Source: CAD feature listing. Evaluate the final solid. Frame: model axes, mm. Give positions to 0.01 mm unless a question says otherwise; leave off trailing zeros. Loops run counter-clockwise (first coordinate to the right, second up) from the corner with the lowest first, then second, coordinate; pieces in that order, holes last. Notation, with made-up numbers: (-12.75, 32.5) -> (28.25, 32.5) arc R35 cw to (28.25, 71.5) -> close; hole circle Ø11 at (-14, 82). An arc over 180 degrees is marked (long way). Answer as a JSON object with one key per item and string values. Group by question number.
from build123d import *

# Parameters (mm, degrees)
F1_W     = 258.840755
F1_H     = 209.543214
F2_DEPTH = 25.4
F3_DEPTH = 25.4
F4_W     = 239.790755
F4_H     = 196.843214
F5_DEPTH = 19.05


with BuildPart() as f2:
    # F1 (on Front) → F2 (new body)
    with BuildSketch(Plane.XZ):
        with Locations((20.0017, 0.897209)):
            Rectangle(F1_W, F1_H)
    extrude(amount=-F2_DEPTH)

    # F0 (on Front) → F3 (cut)
    with BuildSketch(Plane.XZ):
        Polygon((-88.651664, 86.055733), (-82.07436, 74.663833), (-88.651664, 63.271933), (-82.07436, 51.880033), (-88.651664, 40.488133), (-82.07436, 29.096233), (-88.651664, 17.704333), (-82.07436, 6.312433), (-88.651664, -5.079467), (-82.07436, -16.471367), (-88.651664, -27.863267), (-82.07436, -39.255167), (-88.651664, -50.647067), (-82.07436, -62.038967), (-88.651664, -73.430867), (-82.07436, -84.822767), (-68.5546, -84.810067), (-61.977295, -96.201967), (-48.074809, -96.201967), (-41.497504, -84.810067), (-29.09062, -84.810067), (-22.513315, -96.201967), (-8.610829, -96.201967), (-2.033524, -84.810067), (10.37336, -84.810067), (16.950665, -96.201967), (30.853151, -96.201967), (37.430456, -84.810067), (49.83734, -84.810067), (56.414645, -96.201967), (70.308445, -96.201967), (77.259713, -84.162367), (70.682409, -72.770467), (77.259713, -61.378567), (70.682409, -49.986667), (77.259713, -38.594767), (70.682409, -27.202867), (77.259713, -15.810967), (70.682409, -4.419067), (77.259713, 6.972833), (70.682409, 18.364733), (77.259713, 29.756633), (70.682409, 41.148533), (77.259713, 52.540433), (70.682409, 63.932333), (77.259713, 75.324233), (70.681266, 86.718775), (57.162446, 86.703433), (50.585141, 98.095333), (36.682655, 98.095333), (30.10535, 86.703433), (17.698466, 86.703433), (11.121161, 98.095333), (-2.781325, 98.095333), (-9.35863, 86.703433), (-21.765514, 86.703433), (-28.342819, 98.095333), (-42.252925, 98.095333), (-48.83023, 86.703433), (-61.237114, 86.703433), (-67.814419, 98.095333), (-81.700395, 98.095333), align=None)
    extrude(amount=-F3_DEPTH, mode=Mode.SUBTRACT)

    # F4 (on face) → F5 (cut)
    with BuildSketch(Plane(origin=(0, 25.4, 0), x_dir=(-1, 0, 0), z_dir=(0, 1, 0))):
        with Locations((-16.826699, 0.897209)):
            Rectangle(F4_W, F4_H)
    extrude(amount=-F5_DEPTH, mode=Mode.SUBTRACT)


solid = f2.part
(1) Section query A-A on x = -34. Return the cut outline in (y, z), plus the area to 3 significant figures.
(2) Mould query, pull axis X, two halves, no side actions, for faces 1 (the face through (74.02, 3.13, -78.55)), 2 (the face through (73.9, 3.1, -67.2)). Classes: pulls with the +X half, pulls with the -X half, needs draft (parallel to the pull), parting line crosses it, or undercut.
(3) Material intervals for line 1 (X direction, y = 16.5, z = 27); line 2 (Z direction, x = -33, y = 15.25); line 3 (Z direction, x = -76.5, y = 2), sorted ascending. Write a range as from..to.
(4) Section query B-B on z = 55.5. Return the cut outline in (x, y), plus the area to 3 significant figures.
(5) Section query D-D on x = 120. Return the cut outline in (y, z), plus the area to 3 significant figures.
(6) Section query C-C on y = 9.25. Return the cut outline in (x, z).
Result:
{
 "1": {"outline": "(0, -103.87) -> (25.4, -103.87) -> (25.4, -97.52) -> (6.35, -97.52) -> (6.35, -84.81) -> (0, -84.81) -> close; (0, 98.1) -> (6.35, 98.1) -> (6.35, 99.32) -> (25.4, 99.32) -> (25.4, 105.67) -> (0, 105.67) -> close", "area": "411 mm²"},
 "2": {"face 1": "undercut", "face 2": "undercut"},
 "3": {"line 1": "-109.42..-103.07, 136.72..149.42", "line 2": "-103.87..-97.52, 99.32..105.67", "line 3": "-103.87..-84.82, 98.1..105.67"},
 "4": {"outline": "(-109.42, 0) -> (-84.16, 0) -> (-84.16, 6.35) -> (-103.07, 6.35) -> (-103.07, 25.4) -> (-109.42, 25.4) -> close; (75.55, 0) -> (149.42, 0) -> (149.42, 25.4) -> (136.72, 25.4) -> (136.72, 6.35) -> (75.55, 6.35) -> close", "area": "992 mm²"},
 "5": {"outline": "(0, -103.87) -> (25.4, -103.87) -> (25.4, -97.52) -> (6.35, -97.52) -> (6.35, 99.32) -> (25.4, 99.32) -> (25.4, 105.67) -> (0, 105.67) -> close", "area": "1,570 mm²"},
 "6": {"outline": "(-109.42, -103.87) -> (149.42, -103.87) -> (149.42, 105.67) -> (-109.42, 105.67) -> close; hole (-103.07, -97.52) -> (136.72, -97.52) -> (136.72, 99.32) -> (-103.07, 99.32) -> close"}
}
